Design review of the part built by this model. Coordinates are the model's own, in mm. Face numbers are marked on the shaded views. Coordinates: 2 decimals unless noted, no trailing zeros. Loops run counter-clockwise (first coordinate to the right, second up) from the corner with the lowest first, then second, coordinate; pieces in that order, holes last. Notation, with made-up numbers: (63.25, 40.25) -> (87.25, 40.25) arc R16 cw to (87.25, 52.25) -> close; hole circle Ø9 at (38, -9). An arc over 180 degrees is marked (long way). Answer in a Markdown table with one row per item.
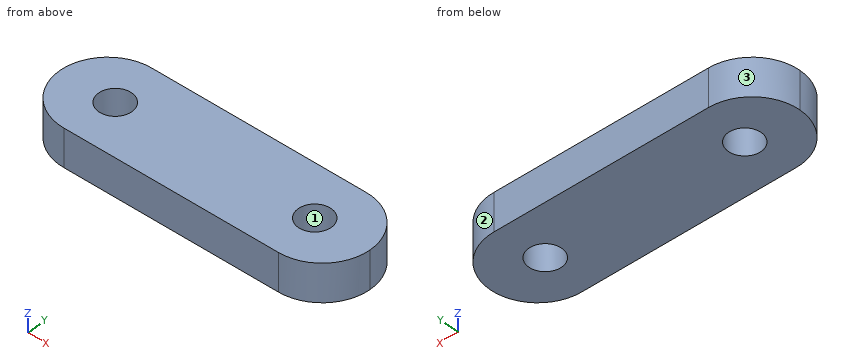
```python
from build123d import *

# Parameters (mm, degrees)
F0_W     = 41.275
F0_H     = 12.7
F1_DEPTH = 5
F2_R     = 2.1845
F2_R_2   = 2.1844
F3_DEPTH = 25
F4_R     = 6.34999


# Not quite as in the source:
# - a fillet or chamfer is up to 0.001 mm smaller than in the source, because OpenCascade refuses the exact size


with BuildPart() as f1:
    # F0 (on Top) → F1 (new body)
    with BuildSketch(Plane.XY):
        with Locations((0.7436354645, -0.3860430318)):
            Rectangle(F0_W, F0_H)
    extrude(amount=F1_DEPTH)

    # F2 (on face) → F3 (cut)
    with BuildSketch(Plane(origin=(0, 0, 0), x_dir=(1, 0, 0), z_dir=(0, 0, -1))):
        with Locations((-12.5438645355, 0.3860430318)):
            Circle(F2_R)
        with Locations((14.0311354645, 0.3860430318)):
            Circle(F2_R_2)
    extrude(amount=-F3_DEPTH, mode=Mode.SUBTRACT)

    # F4 (radius 6.35 in the source; OpenCascade refuses exactly that, so slightly less here)
    f4_edges = [f1.edges().sort_by_distance(p)[0] for p in [
        (21.381135, -6.736043, 2.5),
        (21.381135, 5.963957, 2.5),
        (-19.893865, -6.736043, 2.5),
        (-19.893865, 5.963957, 2.5),
    ]]
    fillet(f4_edges, radius=F4_R)


solid = f1.part
```
(1) Draft analysis for pull direction X (two halves, no side actions). For the marked faces 1, 2 and 3, state which applies: pulls with the +X half, pulls with the -X half, needs draft (parallel to the pull), parting line crosses it, or undercut.
Evaluation:
| item | result |
|---|---|
| face 1 | undercut |
| face 2 | pulls with the +X half |
| face 3 | pulls with the -X half |
(2) For pin 1 (2 mm diameter, centred on y = 0.5, z = 2.5, fed in from +X), flat-tipped, find the tip position at first contact; note if it passes through.
Evaluation:
| item | result |
|---|---|
| pin 1 | stops at x = 21.38 |
(3) Take a section at A-A on z = 0.4. Count the separate pieces of the cut face and the enclosed holes in it, and give its area (3 significant figures).
Evaluation:
| item | result |
|---|---|
| separate pieces | 1 |
| enclosed holes | 2 |
| area | 460 mm² |
(4) Take a section at D-D on y = 4.5. Give the boundary of the cut face in (x, z).
Evaluation:
| item | result |
|---|---|
| outline | (-17.6, 0) -> (19.09, 0) -> (19.09, 5) -> (-17.6, 5) -> close |
(5) Take a section at C-C on x = 15.5. Give the boundary of the cut face in (y, z).
Evaluation:
| item | result |
|---|---|
| outline | (-6.72, 0) -> (-2, 0) -> (-2, 5) -> (-6.72, 5) -> close; (1.23, 0) -> (5.95, 0) -> (5.95, 5) -> (1.23, 5) -> close |
(6) Take a section at B-B on y = -1. Give the boundary of the cut face in (x, z), and give its area (3 significant figures).
Evaluation:
| item | result |
|---|---|
| outline | (-19.86, 0) -> (-14.64, 0) -> (-14.64, 5) -> (-19.86, 5) -> close; (-10.45, 0) -> (11.93, 0) -> (11.93, 5) -> (-10.45, 5) -> close; (16.13, 0) -> (21.35, 0) -> (21.35, 5) -> (16.13, 5) -> close |
| area | 164 mm² |
(7) To check wall thickness, follow probe 1 along X at (y, z) = (1.5, 2.65); probe 2 along X at (y, z) = (-2.25, 0.75); probe 3 along Y at (x, z) = (-13, 4.25). State the ranges of each line that lie inside material, in increasing order.
Evaluation:
| item | result |
|---|---|
| probe 1 | x = -19.61 to -13.65, -11.44 to 12.93, 15.13 to 21.09 |
| probe 2 | x = -19.61 to -13.68, -11.4 to 12.89, 15.17 to 21.1 |
| probe 3 | y = -6.74 to -2.52, 1.75 to 5.96 |
